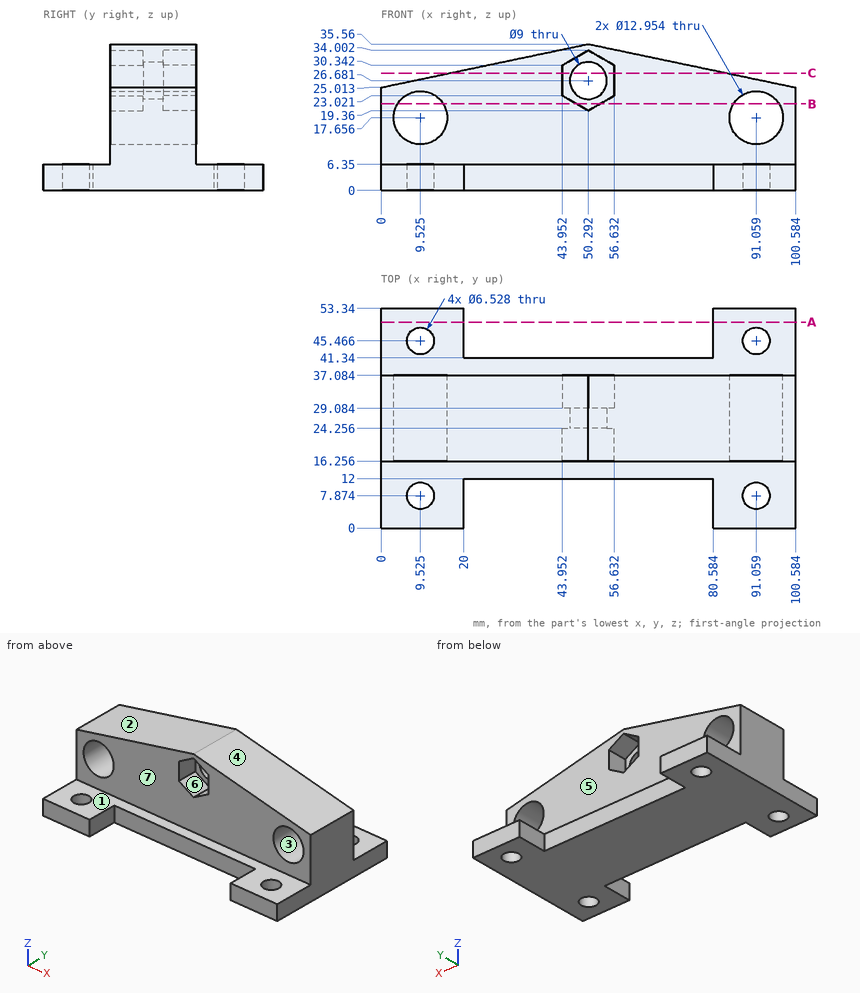
Print and shaded views of the part. All mm, measured from the part's lowest x, y and z. A direction names the side the tool comes from. Round coordinates to 2 decimals unless told otherwise and drop trailing zeros. Write each loop counter-clockwise with the first axis right and the second up, starting at its lowest first coordinate (ties: lowest second). Pieces come first, ordered by that corner, then holes. Notation, with made-up numbers: (72.25, 86) - (88.25, 86) arc R18 cw to (88.25, 115) - close; hole circle Ø9 at (22.25, 3.25). An arc over 180 degrees is marked (long way). One line per item, written item: value.
(1) Wall check: probe 1 along X at (y, z) = (30.5, 22) (1 decimal); probe 2 along Y at (x, z) = (32.5, 27); probe 3 along Z at (x, y) = (19, 13.5). Give the ranges that are in metal, low to high.
Values follow:
probe 1: x = 0 to 4.7, 14.3 to 45.7, 54.9 to 86.3, 95.9 to 100.6
probe 2: y = 16.26 to 37.08
probe 3: z = 0 to 6.35
(2) Cut at C-C, the plane z = 28.5. Give the cut face in (x, y), plus the area to 3 significant figures.
Values follow:
outline: (16.63, 16.26) - (43.95, 16.26) - (43.95, 24.26) - (46.18, 24.26) - (46.18, 29.08) - (43.95, 29.08) - (43.95, 37.08) - (16.63, 37.08) - close; (54.41, 24.26) - (56.63, 24.26) - (56.63, 16.26) - (83.96, 16.26) - (83.96, 37.08) - (56.63, 37.08) - (56.63, 29.08) - (54.41, 29.08) - close
area: 1,160 mm²
(3) 3-axis set-ups, long thin cutter, end or side, ignore diameter. For the marked faces 5, 6 and 7: which of +Z, -Z, +X, -X, +Y, -Y reach the whole face in a straight line?
Values follow:
face 5: +Z, +X, -X, +Y
face 6: -Y
face 7: +Z, +X, -X, -Y
(4) Drop flat-ended pins along their axis: P1, Ø8, axis at x = 24, z = 7.5, coming from the +Y side; P2, Ø3, axis at x = 56.5, z = 18.5, coming from the +Y side; P3, Ø20.5, axis at x = 91.059, z = 17.656, coming from the -Y side. Give the stop position or say it passes through.
Values follow:
P1: stops at y = 41.34
P2: stops at y = 37.08
P3: stops at y = 16.26
(5) Two-plate mould, pull along X, no slides. Class the marked faces 1, 2, 3 and 4: pulls with the +X half, pulls with the -X half, needs draft (parallel to the pull), parting line crosses it, or undercut.
Values follow:
face 1: needs draft
face 2: pulls with the -X half
face 3: undercut
face 4: pulls with the +X half
(6) Cut at A-A, the plane y = 50. Give the cut face in (x, z).
Values follow:
outline: (0, 0) - (20, 0) - (20, 6.35) - (0, 6.35) - close; (80.58, 0) - (100.58, 0) - (100.58, 6.35) - (80.58, 6.35) - close
(7) Cut at B-B, the plane z = 21. Give the cut face in (x, y).
Values follow:
outline: (0, 16.26) - (3.98, 16.26) - (3.98, 37.08) - (0, 37.08) - close; (15.07, 16.26) - (47.45, 16.26) - (47.45, 24.26) - (53.13, 24.26) - (53.13, 16.26) - (85.51, 16.26) - (85.51, 37.08) - (53.13, 37.08) - (53.13, 29.08) - (47.45, 29.08) - (47.45, 37.08) - (15.07, 37.08) - close; (96.61, 16.26) - (100.58, 16.26) - (100.58, 37.08) - (96.61, 37.08) - close
